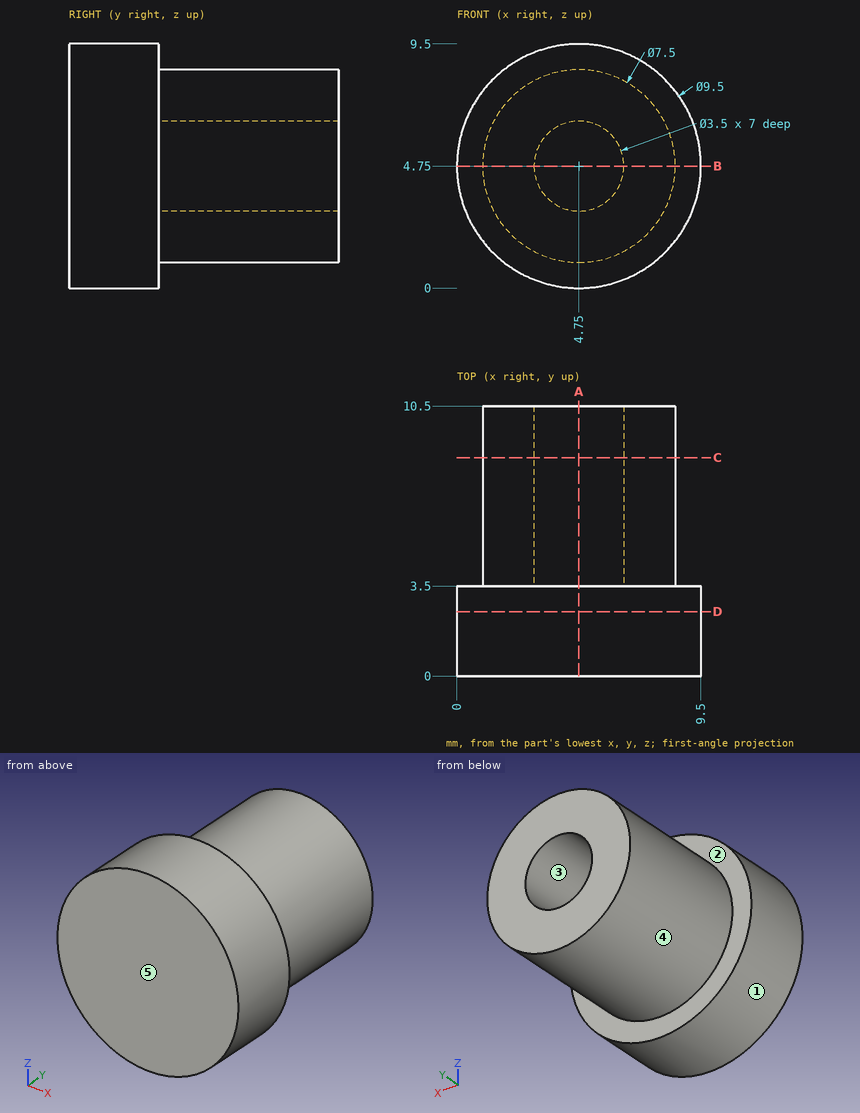
Verification items for this drawing (mm, ordinates from the low corner). A direction names the side the tool comes from. Coordinates: 2 decimals unless noted, no trailing zeros. Order: outer loops, then holes, each group sorted by start corner. A loop starts at its lowest first (then second) coordinate and runs counter-clockwise, first axis right, second up. Notation, with made-up numbers: (80.5, 41) - (139.5, 41) arc R29 ccw to (139.5, 73) - close; hole circle Ø8 at (84, 58.25). An arc over 180 degrees is marked (long way). Answer as a JSON object with one key per item and string values. Group by question number.
Item 1: Sectioned sample at D-D, the plane y = 2.5. Record the cut outline in (x, z), and give its area (3 significant figures).
Item 2: Sectioned sample at B-B, the plane z = 4.75. Record the cut outline in (x, y), and give its area (4 significant figures).
Item 3: Draft check along Z on the marked faces 1, 2 and 3. Enter one of: +Z half, -Z half, draft (parallel to the pull), parting line (faces both ways), or undercut.
Item 4: Sectioned sample at A-A, the plane x = 4.75. Record the cut outline in (y, z), and give its area (4 significant figures).
Item 5: Tool access check on the marked faces 4 and 5. Record the directions out of +Z, -Z, +X, -X, +Y, -Y that give a thin tool (end or side, any length) a straight path to the whole face; none if there is none.
Item 6: Depth check by flat-ended pin: pin 1 Ø1 at (y, z) = (7, 4.5) entering from -X; pin 2 Ø1.5 at (x, y) = (3.5, 7) entering from -Z; pin 3 Ø1.8 at (x, z) = (5, 4.5) entering from +Y. Enter the tip coordinate at first touch or a pass-through.
Item 7: Sectioned sample at C-C, the plane y = 8.5. Record the cut outline in (x, z), and give its area (3 significant figures).
Item 8: Scan lines: probe 1 along X at (y, z) = (8.5, 4.75); probe 2 along Y at (x, z) = (9, 2.75); probe 3 along Z at (x, y) = (4.25, 9.75). Record each from-to range of solid material in increasing order.
Resolved:
{
 "1": {"outline": "circle Ø9.5 at (4.75, 4.75)", "area": "70.9 mm^2"},
 "2": {"outline": "(0, 0) - (9.5, 0) - (9.5, 3.5) - (8.5, 3.5) - (8.5, 10.5) - (6.5, 10.5) - (6.5, 3.5) - (3, 3.5) - (3, 10.5) - (1, 10.5) - (1, 3.5) - (0, 3.5) - close", "area": "61.25 mm^2"},
 "3": {"face 1": "parting line", "face 2": "draft", "face 3": "undercut"},
 "4": {"outline": "(0, 0) - (3.5, 0) - (3.5, 1) - (10.5, 1) - (10.5, 3) - (3.5, 3) - (3.5, 6.5) - (10.5, 6.5) - (10.5, 8.5) - (3.5, 8.5) - (3.5, 9.5) - (0, 9.5) - close", "area": "61.25 mm^2"},
 "5": {"face 4": "+Y", "face 5": "+Z, -Z, +X, -X, -Y"},
 "6": {"pin 1": "x = 1", "pin 2": "z = 1.03", "pin 3": "y = 3.5"},
 "7": {"outline": "circle Ø7.5 at (4.75, 4.75); hole circle Ø3.5 at (4.75, 4.75)", "area": "34.6 mm^2"},
 "8": {"probe 1": "1 to 3, 6.5 to 8.5", "probe 2": "0 to 3.5", "probe 3": "1.03 to 3.07, 6.43 to 8.47"}
}
